Can you work these out from the model? Positions are in its coordinate system, mm. Coordinates: 2 decimals unless noted, no trailing zeros. Answer as a JSON object with one key per item and string values. Group by question number.
from build123d import *

# Parameters (mm, degrees)
F0_W     = 100
F0_H     = 100
F2_W     = 530
F2_H     = 530
F4_T     = -6.35
F5_DEPTH = 25.4


with BuildPart() as f3:
    # F0 (on Top) → F3 section 0
    with BuildSketch(Plane.XY):
        Rectangle(F0_W, F0_H)
    # F2 (on offset) → F3 section 1
    with BuildSketch(Plane.XY.offset(406.66)):
        Rectangle(F2_W, F2_H)
    loft()

    # F4
    f4_openings = [f3.faces().sort_by_distance(p)[0] for p in [
        (0, 0, 406.66),
    ]]
    offset(amount=F4_T, openings=f4_openings)

    # F5 (cut): a face of the model
    f5_faces = [f3.faces().sort_by_distance(p)[0] for p in [
        (0, 0, 0),
    ]]
    extrude(f5_faces, amount=-F5_DEPTH, mode=Mode.SUBTRACT)


solid = f3.part
Q1. Will these pins go through, and if not, where does the flat tip stop? pin 1 (11 mm diameter, centred on y = 12.5, z = 8.5, fed in from +X); pin 2 (1 mm diameter, centred on x = 127, y = -170, fed in from -Z); pin 3 (6 mm diameter, centred on x = 28, y = 168, fed in from +Z).
Q2. We'd pull the mould along Y, two halves only. Please class faces 1 (the flat face through (50, -1, 7)), 2 (the flat face through (-1, 50, 7)): pulls with the +Y half, pulls with the -Y half, needs draft (parallel to the pull), parting line crosses it, or undercut.
Q3. Please list where these lines run through material, in increasing order: L1, parallel to Y at x = -29, z = 111.5; L2, parallel to Y at x = -148, z = 336; L3, parallel to X at y = 17.5, z = 272.
Reply:
{
 "1": {"pin 1": "x = 57.4", "pin 2": "z = 226.03", "pin 3": "z = 242.45"},
 "2": {"face 1": "undercut", "face 2": "undercut"},
 "3": {"L1": "-108.95 to -101.77, 101.77 to 108.95", "L2": "-227.64 to -220.46, 220.46 to 227.64", "L3": "-193.81 to -186.62, 186.62 to 193.81"}
}
